Answer from the drawing. Dimensions are ordinates in mm from the lowest x, y and z of the part. Give positions to 0.01 mm unless a question says otherwise; leave off trailing zeros. Order: outer loops, then holes, each group sorted by start corner. A loop starts at its lowest first (then second) coordinate and runs counter-clockwise, first axis right, second up.
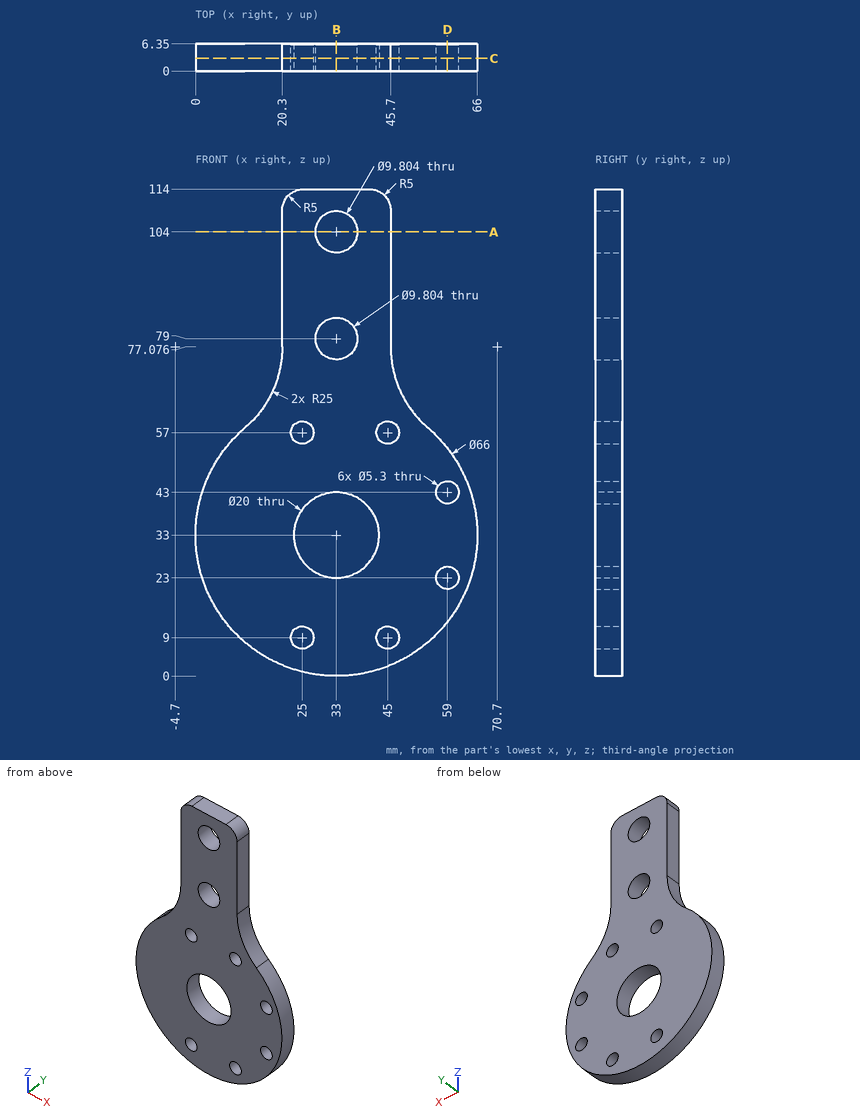
1. The part is cut by section B-B (x = 33). Write down the section's boundary in (y, z).
Findings below:
outline: (0, 0) - (6.35, 0) - (6.35, 23) - (0, 23) - close; (0, 43) - (6.35, 43) - (6.35, 74.1) - (0, 74.1) - close; (0, 83.9) - (6.35, 83.9) - (6.35, 99.1) - (0, 99.1) - close; (0, 108.9) - (6.35, 108.9) - (6.35, 114) - (0, 114) - close
2. Straight lines are drawn through the part: probe 1 along Z at (x, y) = (33, 2.5); probe 2 along Z at (x, y) = (36, 2) (1 decimal); probe 3 along X at (y, z) = (5, 104). For each, find the intervals that lie inside material, in ascending order.
Findings below:
probe 1: z = 0 to 23, 43 to 74.1, 83.9 to 99.1, 108.9 to 114
probe 2: z = 0.1 to 23.5, 42.5 to 75.1, 82.9 to 100.1, 107.9 to 114
probe 3: x = 20.3 to 28.1, 37.9 to 45.7
3. Given P1, Ø1, axis at y = 2, z = 31, coming from the -X side; P2, Ø3, axis at y = 3, z = 93, coming from the -X side; P3, Ø15.5, axis at x = 33, z = 79, coming from the +Y side; P4, Ø1, axis at x = 53.5, y = 2.5, coming from the +Z side, each flat-ended and moving along its own axis, determine where each tip first touches the part or whether it passes through.
Findings below:
P1: stops at x = 0.03
P2: stops at x = 20.3
P3: stops at y = 6.35
P4: stops at z = 59.42
4. The part is cut by section A-A (z = 104). Write down the section's boundary in (x, y).
Findings below:
outline: (20.3, 0) - (28.1, 0) - (28.1, 6.35) - (20.3, 6.35) - close; (37.9, 0) - (45.7, 0) - (45.7, 6.35) - (37.9, 6.35) - close
5. The part is cut by section C-C (y = 3). State how many separate pieces and enclosed holes the cut face has, then the cut area to 3 significant figures.
Findings below:
separate pieces: 1
enclosed holes: 9
area: 4,100 mm2
6. The part is cut by section D-D (x = 59). Write down the section's boundary in (y, z), then the cut area to 3 significant figures.
Findings below:
outline: (0, 12.68) - (6.35, 12.68) - (6.35, 20.35) - (0, 20.35) - close; (0, 25.65) - (6.35, 25.65) - (6.35, 40.35) - (0, 40.35) - close; (0, 45.65) - (6.35, 45.65) - (6.35, 53.32) - (0, 53.32) - close
area: 191 mm2
